```python
from build123d import *

# Parameters (mm, degrees)
BOX001_W            = 10
BOX001_H            = 10
BOX001_DEPTH        = 10
BOX_W               = 7.07
BOX_H               = 10
BOX_DEPTH           = 7.07
BOX_PLACEMENT_ANGLE = 45


with BuildPart() as cubo_base:
    # Box001 → Box001 (new body)
    with BuildSketch(Plane(origin=(-4, -5, 0), x_dir=(1, 0, 0), z_dir=(0, 0, 1))):
        with Locations((5, 5)):
            Rectangle(BOX001_W, BOX001_H)
    extrude(amount=BOX001_DEPTH)


with BuildPart() as fusion:
    # Box → Box (new body)
    with BuildSketch(Plane.XY):
        with Locations((3.535, 5)):
            Rectangle(BOX_W, BOX_H)
    extrude(amount=BOX_DEPTH)


with BuildPart() as fusion_1:
    # Box placement: moved
    add(fusion.part.moved(Location((-4, -5, 10))).rotate(Axis((-4, -5, 10), (0, 1, 0)), BOX_PLACEMENT_ANGLE))

    # Fusion: union cubo_base
    add(cubo_base.part)


solid = fusion_1.part
```
CAD build for the part. Positions are in the model's coordinates, mm. Coordinates: 2 decimals unless noted, no trailing zeros. Write each loop counter-clockwise with the first axis right and the second up, starting at its lowest first coordinate (ties: lowest second). Pieces come first, ordered by that corner, then holes.
(1) Cut at B-B, the plane x = -3. List the corners of the cut face in (y, z).
(2) Cut at C-C, the plane z = 11. List the corners of the cut face in (x, y).
(3) Drill centre lines: probe 1 along Z at (x, y) = (5, -2.75); probe 2 along X at (y, z) = (3.25, 10.75); probe 3 along Z at (x, y) = (-2.5, 0). Where is each one in solid material? Low to high.
Geometry says:
1. outline: (-5, 0) - (5, 0) - (5, 11) - (-5, 11) - close
2. outline: (-3, -5) - (5, -5) - (5, 5) - (-3, 5) - close
3. probe 1: z = 0 to 11
3. probe 2: x = -3.25 to 5.25
3. probe 3: z = 0 to 11.5
